```python
from build123d import *

# Parameters (mm, degrees)
F0_R     = 3.175
F1_DEPTH = 3.048


with BuildPart() as f1:
    # F0 (on Front) → F1 (new body)
    with BuildSketch(Plane.XZ):
        with BuildLine():
            ThreePointArc((-9.525, 114.3), (0, 104.775), (9.525, 114.3))
            ThreePointArc((9.525, 114.3), (0, 123.825), (-9.525, 114.3))
        make_face()
        with Locations((0, 114.3)):
            Circle(F0_R, mode=Mode.SUBTRACT)
        with BuildLine():
            ThreePointArc((-15.747457, 65.508289), (0, 79.375), (15.747457, 65.508289))
            Line((15.747457, 65.508289), (9.525, 114.3))
            ThreePointArc((9.525, 114.3), (0, 104.775), (-9.525, 114.3))
            Line((-9.525, 114.3), (-15.747457, 65.508289))
        make_face()
        with Locations((-3.175, 100.0252)):
            Circle(F0_R, mode=Mode.SUBTRACT)
        with BuildLine():
            ThreePointArc((-15.386538, 59.592308), (1.969051, 47.747589), (15.875, 63.5))
            ThreePointArc((15.875, 63.5), (15.843082, 64.506168), (15.747457, 65.508289))
            ThreePointArc((15.747457, 65.508289), (0, 79.375), (-15.747457, 65.508289))
            ThreePointArc((-15.747457, 65.508289), (-15.843082, 64.506168), (-15.875, 63.5))
            Line((-15.875, 63.5), (-15.386538, 59.592308))
        make_face()
        with Locations((0, 63.5)):
            Circle(F0_R, mode=Mode.SUBTRACT)
        with BuildLine():
            Line((15.875, 15.8877), (15.875, 63.5))
            ThreePointArc((15.875, 63.5), (1.969051, 47.747589), (-15.386538, 59.592308))
            Line((-15.386538, 59.592308), (-7.9375, 0))
            ThreePointArc((-7.9375, 0), (0, 7.9375), (7.9375, 0))
            ThreePointArc((7.9375, 0), (5.61266, -5.61266), (0, -7.9375))
            Line((0, -7.9375), (44.45, -7.9375))
            ThreePointArc((44.45, -7.9375), (36.5125, 0), (44.45, 7.9375))
            Line((44.45, 7.9375), (23.8252, 7.9375))
            ThreePointArc((23.8252, 7.9375), (18.20356, 10.26606), (15.875, 15.8877))
        make_face()
        with BuildLine():
            ThreePointArc((7.9375, 0), (0, 7.9375), (-7.9375, 0))
            ThreePointArc((-7.9375, 0), (-5.61266, -5.61266), (0, -7.9375))
            ThreePointArc((0, -7.9375), (5.61266, -5.61266), (7.9375, 0))
        make_face()
        Circle(F0_R, mode=Mode.SUBTRACT)
        with BuildLine():
            ThreePointArc((52.3875, 0), (50.06266, 5.61266), (44.45, 7.9375))
            ThreePointArc((44.45, 7.9375), (36.5125, 0), (44.45, -7.9375))
            ThreePointArc((44.45, -7.9375), (50.06266, -5.61266), (52.3875, 0))
        make_face()
        with Locations((44.45, 0)):
            Circle(F0_R, mode=Mode.SUBTRACT)
    extrude(amount=-F1_DEPTH)


solid = f1.part
```
Input: part model. Units: mm. Frame: model coordinates. A direction names the side the tool comes from. Give positions to 0.01 mm unless a question says otherwise; leave off trailing zeros. Write each loop counter-clockwise with the first axis right and the second up, starting at its lowest first coordinate (ties: lowest second). Pieces come first, ordered by that corner, then holes. Notation, with made-up numbers: (55, 7.5) - (92, 7.5) arc R7 ccw to (92, 16.5) - close; hole circle Ø9 at (43.5, 76). An arc over 180 degrees is marked (long way). Write item = value, one per line. Start each with the question number.
1. Section query C-C, the plane z = 10.5. Output: boundary loops of the cut face in (x, y).
2. Access query for faces 1 (the cylindrical face through (-3.588, 1.503, 103.173)), 2 (the flat face through (34, 2, 7.938)). Directions: +Z, -Z, +X, -X, +Y, -Y. A direction counts if a zero-diameter tool reaches every point of the face in a straight line with its end or side. Return the directions, or none.
3. Section query B-B, the plane x = 35. Output: boundary loops of the cut face in (y, z).
4. Mould query, pull axis X, two halves, no side actions, for faces 3 (the flat face through (15.875, 2, 39)), 4 (the cylindrical face through (-0.69, 1.5, -3.1)), 5 (the cylindrical face through (-5.674, 1.503, -5.551)), 6 (the cylindrical face through (1.707, 1.503, 66.177)). Classes: released by +X, released by -X, zero draft, split by the parting line, or undercut.
5. Section query A-A, the plane y = 1.8. Count the separate pieces of the cut face and the enclosed holes in it, then the cut area to 3 significant figures.
6. First-contact query: pin 1 Ø0.9 at (y, z) = (2, 45.5) entering from +X (3 decimals). Flat tip, straight axial feed; report the tip coordinate or a pass-through.
7. Ray query, L1, parallel to Z at x = 30, y = 1.4; L2, parallel to X at y = 2.95, z = 61 (1 decimal); L3, parallel to Z at x = 20.5, y = 0.9. Return the intervals inside material, ascending.
Check sheet entries:
q1.outline = (-9.25, 0) - (17.98, 0) - (17.98, 3.05) - (-9.25, 3.05) - close
q2.face_1 = +Y, -Y
q2.face_2 = +Z, +X, +Y, -Y
q3.outline = (0, -7.94) - (3.05, -7.94) - (3.05, 7.94) - (0, 7.94) - close
q4.face_3 = released by +X
q4.face_4 = undercut
q4.face_5 = released by -X
q4.face_6 = undercut
q5.separate_pieces = 1
q5.enclosed_holes = 5
q5.area = 3,790 mm2
q6.pin_1 = 15.875
q7.L1 = -7.94 to 7.94
q7.L2 = -15.6 to -2, 2 to 15.9
q7.L3 = -7.94 to 8.67
